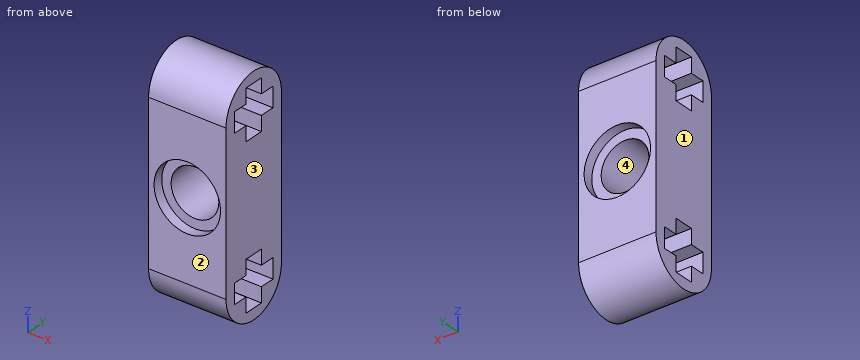
```python
from build123d import *

# Parameters (mm, degrees)
BOSS_EXTRUDE1_DEPTH = 7.8
SKETCH3_R           = 2.4
CUT_EXTRUDE1_DEPTH  = 7.2
SKETCH6_R           = 3.345382302
SKETCH6_R_2         = 2.4
CUT_EXTRUDE3_DEPTH  = 1


with BuildPart() as part:
    # Sketch1 → Boss-Extrude1 (new body)
    with BuildSketch(Plane(origin=(0, 0, 0), x_dir=(0, 0, -1), z_dir=(1, 0, 0))):
        with BuildLine():
            Line((0, -3.6), (-15.9, -3.6))
            ThreePointArc((-15.9, -3.6), (-19.5, 0), (-15.9, 3.6))
            Line((-15.9, 3.6), (0, 3.6))
            ThreePointArc((0, 3.6), (3.6, 0), (0, -3.6))
        make_face()
        Polygon((-2.5, -1), (-1, -1), (-1, -2.5), (1, -2.5), (1, -1), (2.5, -1), (2.5, 1), (1, 1), (1, 2.5), (-1, 2.5), (-1, 1), (-2.5, 1), align=None, mode=Mode.SUBTRACT)
        Polygon((-13.4, -1), (-13.4, 1), (-14.9, 1), (-14.9, 2.5), (-16.9, 2.5), (-16.9, 1), (-18.4, 1), (-18.4, -1), (-16.9, -1), (-16.9, -2.5), (-14.9, -2.5), (-14.9, -1), align=None, mode=Mode.SUBTRACT)
    extrude(amount=BOSS_EXTRUDE1_DEPTH)

    # Sketch3 → Cut-Extrude1 (cut)
    with BuildSketch(Plane(origin=(0, 3.6, 0), x_dir=(1, 0, 0), z_dir=(0, 1, 0))):
        with Locations((3.9, -8)):
            Circle(SKETCH3_R)
    extrude(amount=-CUT_EXTRUDE1_DEPTH, mode=Mode.SUBTRACT)

    # Sketch6 → Cut-Extrude3 (cut)
    with BuildSketch(Plane(origin=(0, 3.6, 0), x_dir=(1, 0, 0), z_dir=(0, 1, 0))):
        with Locations((3.9, -8)):
            Circle(SKETCH6_R)
        with Locations((3.9, -8)):
            Circle(SKETCH6_R_2, mode=Mode.SUBTRACT)
    cut_extrude3 = extrude(amount=-CUT_EXTRUDE3_DEPTH, mode=Mode.SUBTRACT)

    # Mirror1: Cut-Extrude3 across plane
    add(cut_extrude3.mirror(Plane(origin=(0, 0, 0), x_dir=(0, 0, 1), z_dir=(0, -1, 0))), mode=Mode.SUBTRACT)


solid = part.part
```
Geometry check sheet. Reference: the model listing, model coordinates, mm. Face numbers are marked on the shaded views. Coordinates: 2 decimals unless noted, no trailing zeros. Order: outer loops, then holes, each group sorted by start corner. A loop starts at its lowest first (then second) coordinate and runs counter-clockwise, first axis right, second up. Notation, with made-up numbers: (69, 48) - (80, 48) arc R9 cw to (80, 59) - close; hole circle Ø7 at (41, 13). An arc over 180 degrees is marked (long way). Use one line per item in the form item = value.
1. Section check A-A (z = 8). Record the boundary of the cut face in (x, y).
Here are the results:
outline = (0, -3.6) - (0.55, -3.6) - (0.55, -2.6) - (1.5, -2.6) - (1.5, 2.6) - (0.55, 2.6) - (0.55, 3.6) - (0, 3.6) - close; (6.3, -2.6) - (7.25, -2.6) - (7.25, -3.6) - (7.8, -3.6) - (7.8, 3.6) - (7.25, 3.6) - (7.25, 2.6) - (6.3, 2.6) - close
2. Draft check along X on the marked faces 1, 2, 3 and 4. Enter one of: pulls with the +X half, pulls with the -X half, needs draft (parallel to the pull), parting line crosses it, or undercut.
Here are the results:
face_1 = pulls with the -X half
face_2 = needs draft
face_3 = pulls with the +X half
face_4 = undercut
3. Section check B-B (y = 0). Record the boundary of the cut face in (x, z), then the cut area to 3 significant figures.
Here are the results:
outline = (0, -3.6) - (7.8, -3.6) - (7.8, -2.5) - (0, -2.5) - close; (0, 2.5) - (7.8, 2.5) - (7.8, 13.4) - (0, 13.4) - close; (0, 18.4) - (7.8, 18.4) - (7.8, 19.5) - (0, 19.5) - close; hole circle Ø4.8 at (3.9, 8)
area = 84.1 mm²
4. Scan lines: line 1 (X direction, y = 2.95, z = 8); line 2 (Z direction, x = 4, y = 0.25); line 3 (X direction, y = 0.6, z = 8). Record each from-to range of solid material in increasing order.
Here are the results:
line_1 = 0 to 0.55, 7.25 to 7.8
line_2 = -3.59 to -2.5, 2.5 to 5.6, 10.4 to 13.4, 18.4 to 19.49
line_3 = 0 to 1.5, 6.3 to 7.8
5. Section check D-D (y = 1.5). Record the boundary of the cut face in (x, z), then the cut area to 3 significant figures.
Here are the results:
outline = (0, -3.27) - (7.8, -3.27) - (7.8, -1) - (0, -1) - close; (0, 1) - (7.8, 1) - (7.8, 14.9) - (0, 14.9) - close; (0, 16.9) - (7.8, 16.9) - (7.8, 19.17) - (0, 19.17) - close; hole circle Ø4.8 at (3.9, 8)
area = 126 mm²
6. Gauge pin test, flat ends, axial feed: pin 1 (1.2 mm diameter, centred on x = 2.5, y = 1.5, fed in from +Z); pin 2 (1.6 mm diameter, centred on x = 5.5, y = 2, fed in from +Z); pin 3 (1 mm diameter, centred on x = 5, y = 2, fed in from -Z). Record the tip position at first contact, or that the pin passes through.
Here are the results:
pin_1 = 19.39
pin_2 = 19.29
pin_3 = -3.27
7. Section check C-C (x = 3.9). State how many separate pieces and enclosed holes the cut face has, then the cut area to 3 significant figures.
Here are the results:
separate_pieces = 2
enclosed_holes = 2
area = 84.9 mm²
